Design review of the part built by this model. Coordinates are the model's own, in mm. A direction names the side the tool comes from. Give positions to 0.01 mm unless a question says otherwise; leave off trailing zeros. Loops run counter-clockwise (first coordinate to the right, second up) from the corner with the lowest first, then second, coordinate; pieces in that order, holes last.
from build123d import *

# Parameters (mm, degrees)
F2_R     = 3.175
F4_R     = 2.54
F5_W     = 34.6189280972
F5_H     = 141.0606596619
F6_DEPTH = 25.4


with BuildPart() as f3:
    # F3: sweep along a path in F0
    with BuildLine(Plane.XZ) as f3_path:
        ThreePointArc((50.8, -76.2), (25.4, -101.6), (0, -76.2))
        Line((0, -76.2), (0, 0))
    # F2 (on plane+point) → F3 (sweep)
    with BuildSketch(Plane.XY.offset(-76.2)):
        with Locations((50.8, 0)):
            Circle(F2_R)
    sweep(path=f3_path.line)

    # F4
    f4_edges = [f3.edges().sort_by_distance(p)[0] for p in [
        (47.625, 0, -76.2),
    ]]
    fillet(f4_edges, radius=F4_R)

    # F5 (on Right) → F6 (cut)
    with BuildSketch(Plane.YZ):
        with Locations((-2.6043397374, -54.7910733148)):
            Rectangle(F5_W, F5_H)
    extrude(amount=-F6_DEPTH, mode=Mode.SUBTRACT)


solid = f3.part
Q1. Tool access review of faces 1 (the face through (1, 0, 0)), 2 (the face through (3.174, -0.07, -37.567)): name each direction out of +Z, -Z, +X, -X, +Y, -Y from which nothing blocks a thin tool from reaching the whole face with its end or side.
Results:
face 1: +Z, +X, -X, +Y, -Y
face 2: +Z, +X
Q2. Take a section at A-A (z = -6.5). Give the boundary of the cut face in (x, y) (3 decimals).
Results:
outline: (0, -3.175) arc R3.175 ccw to (0, 3.175) - close
Q3. Wall thickness on line 1 (X direction, y = -1.75, z = -85); line 2 (X direction, y = 0.25, z = -39); line 3 (X direction, y = 2.25, z = -86): over which ranges is each line inside the solid? List them lowest first.
Results:
line 1: x = 0 to 4.42, 46.38 to 52.03
line 2: x = 0 to 3.17
line 3: x = 0 to 4.42, 46.38 to 51.24
Q4. Insertion check: pin 1 (1.5 mm diameter, centred on x = 15, y = 0.5, fed in from -Z); pin 2 (0.6 mm diameter, centred on x = 50.5, y = 0, fed in from +Z); pin 3 (1 mm diameter, centred on x = 7.5, y = 1, fed in from +Z). Each pin has a flat end and moves straight along its axis. Give the tip position at first contact, or say it passes through.
Results:
pin 1: stops at z = -103.07
pin 2: stops at z = -76.2
pin 3: stops at z = -88.9
